Could you check a few things on this model? Use its own coordinates, in mm. A direction names the side the tool comes from. Round coordinates to 2 decimals unless told otherwise and drop trailing zeros. Loops run counter-clockwise (first coordinate to the right, second up) from the corner with the lowest first, then second, coordinate; pieces in that order, holes last. Notation, with made-up numbers: (17, 68.5) -> (52, 68.5) arc R28 ccw to (52, 92.5) -> close; hole circle Ø6 at (-19.75, 8.25). An arc over 180 degrees is marked (long way). Put each result on its own line as item: value. Start each with the question number.
1. Imagine slicing it at D-D, the plane y = -93. Please give me the cut outline in (x, z), and give its area (3 significant figures).
2. I need wall thicknesses on line 1 (X direction, y = -16, z = 2.2); line 2 (Y direction, x = 45.5, z = 1.3); line 3 (X direction, y = -66, z = 1.75). Which ranges of each line are inside material? Lowest first, please. Write a range as [from, to].
3. If we mould it in two halves opening along X, with no side actions, what happens to faces 3 (the flat face through (33, 28, 0)), 4 (the flat face through (-71.829, 89.556, 1.479)), 5 (the cylindrical face through (-31.59, 38.84, 1.48))? For each: pulls with the +X half, pulls with the -X half, needs draft (parallel to the pull), parting line crosses it, or undercut.
4. Imagine slicing it at B-B, the plane z = 0.5. Please give me the cut outline in (x, y).
5. Imagine slicing it at C-C, the plane x = 90. Please give me the cut outline in (y, z), and give its area (3 significant figures).
6. Imagine slicing it at A-A, the plane y = 11. Please give me the cut outline in (x, z).
7. Which directions (+Z, -Z, +X, -X, +Y, -Y) give clear straight access to the entire face, cutting with the end or side of a thin tool? Please do faces 1 (the flat face through (33, 28, 3)), 2 (the cylindrical face through (-79.9, 38.5, 1.5)).
8. I'm going to push flat-ended pins straight in: P1, Ø6, axis at x = -38.5, y = 57, coming from the -Z side; P2, Ø1.5, axis at x = -51.5, z = 2, coming from the -Y side. Where does each tip first touch, or does it pass through?
```python
from build123d import *

# Parameters (mm, degrees)
F1_DEPTH = 3


with BuildPart() as f1:
    # F0 (on Top) → F1 (new body)
    with BuildSketch(Plane.XY):
        with BuildLine():
            Line((-34.152171, 123.5992), (-110.575682, 54.545258))
            Line((-110.575682, 54.545258), (-110.575682, -125.454742))
            Line((-110.575682, -125.454742), (-85.575682, -125.454742))
            Line((-85.575682, -125.454742), (-85.575682, 24.545258))
            ThreePointArc((-85.575682, 24.545258), (-79.717818, 38.687394), (-65.575682, 44.545258))
            Line((-65.575682, 44.545258), (-45.575682, 44.545258))
            ThreePointArc((-45.575682, 44.545258), (-31.433547, 38.687394), (-25.575682, 24.545258))
            Line((-25.575682, 24.545258), (-25.575682, -59.4008))
            Line((-25.575682, -59.4008), (180.847829, -59.4008))
            Line((180.847829, -59.4008), (180.847829, 123.5992))
            Line((180.847829, 123.5992), (-34.152171, 123.5992))
        make_face()
    extrude(amount=F1_DEPTH)


solid = f1.part
```
Entries:
1. outline: (-110.58, 0) -> (-85.58, 0) -> (-85.58, 3) -> (-110.58, 3) -> close
1. area: 75.0 mm^2
2. line 1: [-110.58, -85.58], [-25.58, 180.85]
2. line 2: [-59.4, 123.6]
2. line 3: [-110.58, -85.58]
3. face 3: needs draft
3. face 4: pulls with the -X half
3. face 5: undercut
4. outline: (-110.58, -125.45) -> (-85.58, -125.45) -> (-85.58, 24.55) arc R20 cw to (-65.58, 44.55) -> (-45.58, 44.55) arc R20 cw to (-25.58, 24.55) -> (-25.58, -59.4) -> (180.85, -59.4) -> (180.85, 123.6) -> (-34.15, 123.6) -> (-110.58, 54.55) -> close
5. outline: (-59.4, 0) -> (123.6, 0) -> (123.6, 3) -> (-59.4, 3) -> close
5. area: 549 mm^2
6. outline: (-110.58, 0) -> (-85.58, 0) -> (-85.58, 3) -> (-110.58, 3) -> close; (-25.58, 0) -> (180.85, 0) -> (180.85, 3) -> (-25.58, 3) -> close
7. face 1: +Z, +X, -X, +Y, -Y
7. face 2: +Z, -Z, -Y
8. P1: z = 0
8. P2: y = 44.55
